from build123d import *

# Parameters (mm, degrees)
PAD_DEPTH            = 20
SKETCH001_W          = 18
SKETCH001_H          = 16
POCKET_DEPTH         = 18.001
POCKET001_DEPTH      = 2.001
POCKET002_DEPTH      = 1
POCKET002_DEPTH_BACK = -5
POCKET003_DEPTH      = 2.001
POCKET004_DEPTH      = 1


with BuildPart() as part:
    # Sketch → Pad (new body)
    with BuildSketch(Plane.XY):
        Polygon((0, 0), (0, 20), (20, 0), align=None)
    extrude(amount=PAD_DEPTH)

    # Sketch001 → Pocket (cut, through all)
    with BuildSketch(Plane.XZ.offset(-2)):
        with Locations((11, 10)):
            Rectangle(SKETCH001_W, SKETCH001_H)
    extrude(amount=-POCKET_DEPTH, mode=Mode.SUBTRACT)

    # Sketch002 (on Face9 of Pocket) → Pocket001 (cut, through all)
    with BuildSketch(Plane.YZ.offset(2)):
        with BuildLine():
            ThreePointArc((4.8, 12.8), (2, 10), (4.8, 7.2))
            Line((4.8, 7.2), (15.2, 7.2))
            ThreePointArc((15.2, 7.2), (18, 10), (15.2, 12.8))
            Line((4.8, 12.8), (15.2, 12.8))
        make_face()
    extrude(amount=-POCKET001_DEPTH, mode=Mode.SUBTRACT)

    # Sketch003 (on Face13 of Pocket001) → Pocket002 (cut, two sides)
    with BuildSketch(Plane.YZ.offset(2)) as pocket002_sk:
        with BuildLine():
            ThreePointArc((15.2, 5.5), (19.7, 10), (15.2, 14.5))
            Line((4.8, 14.5), (15.2, 14.5))
            ThreePointArc((4.8, 14.5), (3.317186, 14.248678), (2, 13.522783))
            Line((2, 13.522783), (2, 6.477217))
            ThreePointArc((2, 6.477217), (3.317186, 5.751322), (4.8, 5.5))
            Line((4.8, 5.5), (15.2, 5.5))
        make_face()
    extrude(amount=-POCKET002_DEPTH, mode=Mode.SUBTRACT)
    extrude(pocket002_sk.sketch, amount=-POCKET002_DEPTH_BACK, mode=Mode.SUBTRACT)

    # Sketch004 (on Face21 of Pocket002) → Pocket003 (cut, through all)
    with BuildSketch(Plane(origin=(0, 2, 0), x_dir=(-1, 0, 0), z_dir=(0, 1, 0))):
        with BuildLine():
            ThreePointArc((-15.2, 12.8), (-18, 10), (-15.2, 7.2))
            Line((-15.2, 7.2), (-4.8, 7.2))
            ThreePointArc((-4.8, 7.2), (-2, 10), (-4.8, 12.8))
            Line((-15.2, 12.8), (-4.8, 12.8))
        make_face()
    extrude(amount=-POCKET003_DEPTH, mode=Mode.SUBTRACT)

    # Sketch005 (on Face15 of Pocket003) → Pocket004 (cut)
    with BuildSketch(Plane(origin=(0, 2, 0), x_dir=(-1, 0, 0), z_dir=(0, 1, 0))):
        with BuildLine():
            ThreePointArc((-15.2, 14.5), (-19.7, 10), (-15.2, 5.5))
            Line((-15.2, 5.5), (-4.8, 5.5))
            ThreePointArc((-4.8, 5.5), (-3.317186, 5.751322), (-2, 6.477217))
            Line((-2, 13.522783), (-2, 6.477217))
            ThreePointArc((-2, 13.522783), (-3.317186, 14.248678), (-4.8, 14.5))
            Line((-15.2, 14.5), (-4.8, 14.5))
        make_face()
    extrude(amount=-POCKET004_DEPTH, mode=Mode.SUBTRACT)


solid = part.part
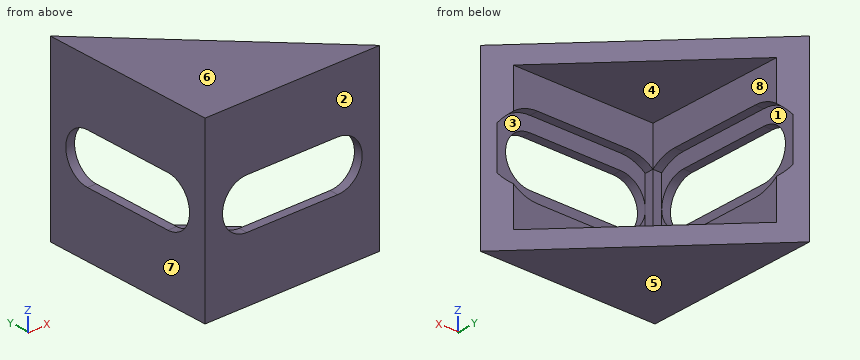
Design review of the part built by this model. Coordinates are the model's own, in mm. Face numbers are marked on the shaded views. A direction names the side the tool comes from. Coordinates: 2 decimals unless noted, no trailing zeros. Loops run counter-clockwise (first coordinate to the right, second up) from the corner with the lowest first, then second, coordinate; pieces in that order, holes last. Notation, with made-up numbers: (85, -9) -> (117, -9) arc R30 ccw to (117, 25) -> close; hole circle Ø1 at (65.5, 1.25). An arc over 180 degrees is marked (long way). Use a Markdown table: item, result. Add a question column.
Item 1: We need section B-B, the plane x = 11. Write out the cut boundary in (y, z), and give its area (3 significant figures).
Item 2: Machinability: for the marked faces 1, 2, 3 and 4, which of the approach directions +Z, -Z, +X, -X, +Y, -Y give a long, thin tool a straight path to every point of the face, cutting with its end or side? Answer none if there is none.
Item 3: We need section A-A, the plane y = 7. Write out the cut boundary in (x, z), and give its area (3 significant figures).
Item 4: The part is to be moulded in two halves that separate along Z. For the marked faces 5, 6, 7 and 8, say which applies: +Z half, -Z half, draft (parallel to the pull), parting line (faces both ways), or undercut.
Item 5: Clearance check with flat-ended pins moving along their axes: P1, Ø8, axis at x = 7.5, z = 5, coming from the +Y side; P2, Ø4, axis at x = 8, z = 15, coming from the +Y side; P3, Ø10, axis at y = 9, z = 8.5, coming from the +X side. State where each tip first meets the part, or that it passes through.
Item 6: Wall thickness on L1, parallel to Z at x = 4, y = 13.75; L2, parallel to Z at x = 1.25, y = 6.5; L3, parallel to Y at x = 14.75, z = 17.75: over which ranges is each line inside the solid? List them lowest first. Write a range as from..to.
Item 7: We need section C-C, the plane y = 18.5. Write out the cut boundary in (x, z), and give its area (3 significant figures).
Item 8: We need section D-D, the plane z = 1.5. Write out the cut boundary in (x, y).
Numbers:
| question | item | result |
|---|---|---|
| 1 | outline | (0, 0) -> (9, 0) -> (9, 2) -> (2, 2) -> (2, 5.5) -> (1, 5.5) -> (1, 7.2) -> (0, 7.2) -> close; (0, 12.8) -> (1, 12.8) -> (1, 14.5) -> (2, 14.5) -> (2, 18) -> (9, 18) -> (9, 20) -> (0, 20) -> close |
| 1 | area | 53.4 mm^2 |
| 2 | face 1 | +X |
| 2 | face 2 | +Z, -Z, +X, -X, -Y |
| 2 | face 3 | +Y |
| 2 | face 4 | +X, +Y |
| 3 | outline | (0, 0) -> (13, 0) -> (13, 2) -> (2, 2) -> (2, 5.5) -> (1, 5.5) -> (1, 7.2) -> (0, 7.2) -> close; (0, 12.8) -> (1, 12.8) -> (1, 14.5) -> (2, 14.5) -> (2, 18) -> (13, 18) -> (13, 20) -> (0, 20) -> close |
| 3 | area | 69.4 mm^2 |
| 4 | face 5 | -Z half |
| 4 | face 6 | +Z half |
| 4 | face 7 | draft |
| 4 | face 8 | undercut |
| 5 | P1 | stops at y = 15.15 |
| 5 | P2 | stops at y = 2 |
| 5 | P3 | stops at x = 2 |
| 6 | L1 | z = 0..2, 18..20 |
| 6 | L2 | z = 0..5.5, 14.5..20 |
| 6 | L3 | y = 0..2 |
| 7 | outline | (0, 0) -> (1.5, 0) -> (1.5, 6.94) -> (1, 6.94) -> (1, 13.06) -> (1.5, 13.06) -> (1.5, 20) -> (0, 20) -> close |
| 7 | area | 26.9 mm^2 |
| 8 | outline | (0, 0) -> (20, 0) -> (0, 20) -> close |
